Build history of the part. All positions in model axes, mm. Face numbers are marked on the shaded views. A direction names the side the tool comes from. Give positions to 0.01 mm unless a question says otherwise; leave off trailing zeros. Order: outer loops, then holes, each group sorted by start corner. A loop starts at its lowest first (then second) coordinate and runs counter-clockwise, first axis right, second up. Notation, with made-up numbers: (23.5, -32) -> (54.5, -32) arc R4 cw to (54.5, -26) -> close; hole circle Ø1 at (-17, 21). An arc over 180 degrees is marked (long way). One line per item, written item: value. Start each with the question number.
(1) Which spindle directions (+Z, -Z, +X, -X, +Y, -Y) get a long thin tool onto all of the face, cutting with end or side? Do the marked faces 1 and 2. Say none if no direction does.
(2) Pin check, flat tips, straight feed: pin 1 (3.5 mm diameter, centred on x = 1.5, z = 7.5, fed in from +Y); pin 2 (2.5 mm diameter, centred on x = 20, y = 48, fed in from +Z); pin 3 (8 mm diameter, centred on x = -16.5, y = 22.5, fed in from +Z). Stop position of each tip, or through.
(3) Probe line 1 (X direction, y = 0.7, z = 7.5); line 2 (X direction, y = 1.95, z = 1.5); line 3 (Z direction, x = -0.5, y = 21.5). List the from-to ranges inside material, lowest first.
(4) Saw through at D-D on y = 48. Give the cut face in (x, z), plus the area to 3 significant figures.
(5) Saw through at B-B on x = 20. Give the cut face in (y, z).
(6) Saw through at C-C on z = -8.5. Give the cut face in (x, y), plus the area to 3 significant figures.
(7) Saw through at A-A on z = 7.5. Give the cut face in (x, y).
```python
from build123d import *

# Parameters (mm, degrees)
SKETCH1_W           = 50
SKETCH1_H           = 45
BOSS_EXTRUDE1_DEPTH = 3
SKETCH2_W           = 50
SKETCH2_H           = 3
BOSS_EXTRUDE2_DEPTH = 50
SKETCH3_R           = 1.6
SKETCH3_R_2         = 1.1
CUT_EXTRUDE1_DEPTH  = 3
SKETCH4_R           = 1.6
CUT_EXTRUDE2_DEPTH  = 3
FILLET1_R           = 4
FILLET2_R           = 3
FILLET3_R           = 6


with BuildPart() as part:
    # Sketch1 → Boss-Extrude1 (new body)
    with BuildSketch(Plane(origin=(0, 0, 0), x_dir=(1, 0, 0), z_dir=(0, 1, 0))):
        Rectangle(SKETCH1_W, SKETCH1_H)
    extrude(amount=BOSS_EXTRUDE1_DEPTH)

    # Sketch2 → Boss-Extrude2 (add)
    with BuildSketch(Plane(origin=(0, 3, 0), x_dir=(1, 0, 0), z_dir=(0, 1, 0))):
        with Locations((0, 21)):
            Rectangle(SKETCH2_W, SKETCH2_H)
    extrude(amount=BOSS_EXTRUDE2_DEPTH)

    # Sketch3 → Cut-Extrude1 (cut)
    with BuildSketch(Plane(origin=(0, 3, 0), x_dir=(1, 0, 0), z_dir=(0, 1, 0))):
        with Locations(Location((3, 8.5, 0), (0, 0, 270))):
            Circle(SKETCH3_R)
        with Locations(Location((3, -11.5, 0), (0, 0, 90))):
            Circle(SKETCH3_R)
        with Locations(Location((-20.7, -1.5, 0), (0, 0, 270))):
            Circle(SKETCH3_R)
        with Locations(Location((1.5, 4.5, 0), (0, 0, 270))):
            Circle(SKETCH3_R_2)
        with Locations(Location((1.5, -7.5, 0), (0, 0, 90))):
            Circle(SKETCH3_R_2)
        with Locations(Location((-20.5, 4.5, 0), (0, 0, 270))):
            Circle(SKETCH3_R_2)
        with Locations(Location((-20.5, -7.5, 0), (0, 0, 90))):
            Circle(SKETCH3_R_2)
    extrude(amount=-CUT_EXTRUDE1_DEPTH, mode=Mode.SUBTRACT)

    # Sketch4 → Cut-Extrude2 (cut)
    with BuildSketch(Plane.XY.offset(-19.5)):
        with Locations((-20, 48)):
            Circle(SKETCH4_R)
        with Locations((20, 48)):
            Circle(SKETCH4_R)
        with Locations((20, 8)):
            Circle(SKETCH4_R)
        with Locations((-20, 8)):
            Circle(SKETCH4_R)
        with Locations((0, 28)):
            Circle(SKETCH4_R)
    extrude(amount=-CUT_EXTRUDE2_DEPTH, mode=Mode.SUBTRACT)

    # Fillet1
    fillet1_edges = [part.edges().sort_by_distance(p)[0] for p in [
        (-25, 53, -21),
        (25, 53, -21),
        (25, 1.5, 22.5),
        (-25, 1.5, 22.5),
    ]]
    fillet(fillet1_edges, radius=FILLET1_R)

    # Fillet2
    fillet2_edges = [part.edges().sort_by_distance(p)[0] for p in [
        (0, 3, -19.5),
    ]]
    fillet(fillet2_edges, radius=FILLET2_R)

    # Fillet3
    fillet3_edges = [part.edges().sort_by_distance(p)[0] for p in [
        (0, 0, -22.5),
    ]]
    fillet(fillet3_edges, radius=FILLET3_R)


solid = part.part
```
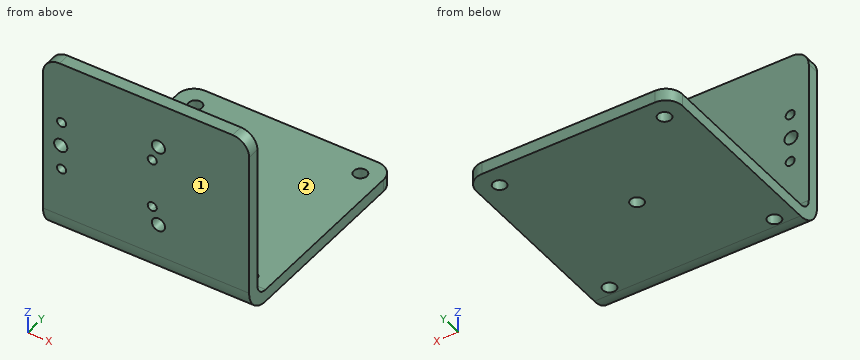
Results below:
1. face 1: +Z, -Z, +X, -X, -Y
1. face 2: +Z, +X, -X, +Y
2. pin 1: stops at y = 3
2. pin 2: passes through
2. pin 3: stops at z = -19.5
3. line 1: x = -25 to -21.6, -19.4 to 0.4, 2.6 to 25
3. line 2: x = -25 to -22.3, -19.1 to 25
3. line 3: z = -22.5 to -19.5
4. outline: (-25, -22.5) -> (-21.6, -22.5) -> (-21.6, -19.5) -> (-25, -19.5) -> close; (-18.4, -22.5) -> (18.4, -22.5) -> (18.4, -19.5) -> (-18.4, -19.5) -> close; (21.6, -22.5) -> (25, -22.5) -> (25, -19.5) -> (21.6, -19.5) -> close
4. area: 131 mm²
5. outline: (0, -16.5) arc R6 ccw to (6, -22.5) -> (6.4, -22.5) -> (6.4, -19.5) -> (6, -19.5) arc R3 cw to (3, -16.5) -> (3, 22.5) -> (0, 22.5) -> close; (9.6, -22.5) -> (46.4, -22.5) -> (46.4, -19.5) -> (9.6, -19.5) -> close; (49.6, -22.5) -> (53, -22.5) -> (53, -19.5) -> (49.6, -19.5) -> close
6. outline: (-25, 0) -> (1.4, 0) -> (1.4, 3) -> (-25, 3) -> close; (4.6, 0) -> (25, 0) -> (25, 3) -> (4.6, 3) -> close
6. area: 140 mm²
7. outline: (-25, 0) -> (-21.6, 0) -> (-21.6, 3) -> (-25, 3) -> close; (-19.4, 0) -> (0.4, 0) -> (0.4, 3) -> (-19.4, 3) -> close; (2.6, 0) -> (25, 0) -> (25, 3) -> (2.6, 3) -> close
